Read the model definition and answer for the solid it produces. Units are mm, in the model's axes. Face numbers are marked on the shaded views. Give positions to 0.01 mm unless a question says otherwise; leave off trailing zeros. Loops run counter-clockwise (first coordinate to the right, second up) from the corner with the lowest first, then second, coordinate; pieces in that order, holes last.
(1) Determine the mould class of the marked faces 1 and 2 for opening direction X: pulls with the +X half, pulls with the -X half, needs draft (parallel to the pull), parting line crosses it, or undercut.
(2) Find section A-A, the plane x = 0. Write down the section's boundary in (y, z).
(3) Find section B-B, the plane y = 34. Write down the section's boundary in (x, z).
(4) Straight lines are drawn through the part: probe 1 along Y at (x, z) = (-5.5, 15.5); probe 2 along Y at (x, z) = (-3.5, -3); probe 3 along Y at (x, z) = (13, -24.5). For each, find the intervals that lie inside material, in ascending order.
(5) Each of these flat-tipped pins is pushed along its axis until it touches: P1, Ø10.5, axis at x = 6, z = 0, coming from the -Y side; P2, Ø3, axis at x = -19, y = -20.5, coming from the -Z side; P3, Ø6, axis at x = -2, y = 187.5, coming from the +Z side. Where does it stop, or does it pass through?
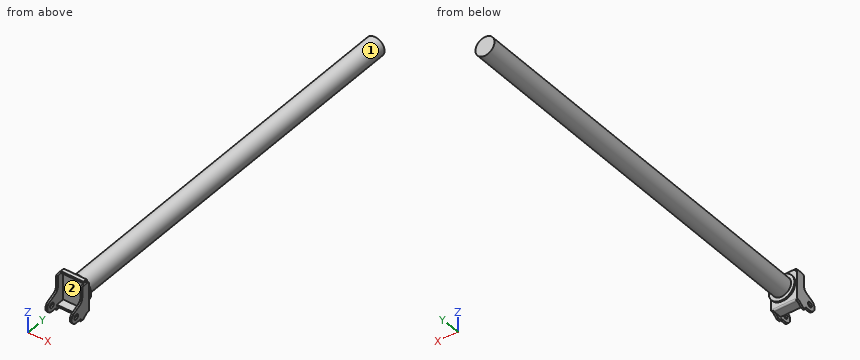
```python
from build123d import *

# Parameters (mm, degrees)
SKETCH1_W           = 35.2425
SKETCH1_H           = 45.085
BOSS_EXTRUDE1_DEPTH = 2.794
SKETCH3_W           = 35.2425
SKETCH3_H           = 7.62
BOSS_EXTRUDE2_DEPTH = 2.794
SKETCH4_W           = 35.2425
SKETCH4_H           = 15.875
BOSS_EXTRUDE3_DEPTH = 2.794
SKETCH5_R           = 3.99415
BOSS_EXTRUDE5_DEPTH = 2.794
SKETCH8_R           = 14.8209
BOSS_EXTRUDE6_DEPTH = 609.6
FILLET1_R           = 2.54


with BuildPart() as part:
    # Sketch1 → Boss-Extrude1 (new body)
    with BuildSketch(Plane(origin=(0, 0, 0), x_dir=(1, 0, 0), z_dir=(0, 1, 0))):
        Rectangle(SKETCH1_W, SKETCH1_H)
    extrude(amount=BOSS_EXTRUDE1_DEPTH)

    # Sketch3 → Boss-Extrude2 (add)
    with BuildSketch(Plane.XY.offset(22.5425)):
        with Locations((0, -1.016)):
            Rectangle(SKETCH3_W, SKETCH3_H)
    extrude(amount=BOSS_EXTRUDE2_DEPTH)

    # Sketch4 → Boss-Extrude3 (add)
    with BuildSketch(Plane(origin=(0, 0, -22.5425), x_dir=(-1, 0, 0), z_dir=(0, 0, -1))):
        with Locations((0, -5.1435)):
            Rectangle(SKETCH4_W, SKETCH4_H)
    extrude(amount=BOSS_EXTRUDE3_DEPTH)

    # Sketch5 → Boss-Extrude5 (add)
    with BuildSketch(Plane.ZY.offset(17.62125)):
        with BuildLine():
            Line((-24.5745, 2.794), (-24.5745, -0.249652205))
            ThreePointArc((-24.5745, -0.249652205), (-24.707295287, -1.060186269), (-25.091795645, -1.785968283))
            Line((-25.091795645, -1.785968283), (-30.3911, -8.763))
            Line((-30.3911, -8.763), (-30.3911, -13.843))
            Line((-30.3911, -13.843), (-26.9875, -13.843))
            Line((-26.9875, -13.843), (-26.9875, -23.3045))
            ThreePointArc((-26.9875, -23.3045), (-19.506235123, -32.571845213), (-8.869629771, -27.213147793))
            Line((-8.869629771, -27.213147793), (-4.188060723, -16.867828085))
            ThreePointArc((-4.188060723, -16.867828085), (-0.439339327, -12.518932794), (5.068277097, -10.8966))
            Line((5.068277097, -10.8966), (19.5707, -10.8966))
            ThreePointArc((19.5707, -10.8966), (21.366751224, -10.152651224), (22.1107, -8.3566))
            Line((22.1107, -8.3566), (22.1107, 0.254))
            ThreePointArc((22.1107, 0.254), (21.366751224, 2.050051224), (19.5707, 2.794))
            Line((19.5707, 2.794), (-24.5745, 2.794))
        make_face()
        with Locations((-17.50695, -23.3045)):
            Circle(SKETCH5_R, mode=Mode.SUBTRACT)
    boss_extrude5 = extrude(amount=BOSS_EXTRUDE5_DEPTH)

    # Mirror1: Boss-Extrude5 across plane
    add(boss_extrude5.mirror(Plane(origin=(0, 0, 0), x_dir=(0, 0, 1), z_dir=(1, 0, 0))))

    # Sketch6 → Revolve1 (revolve)
    with BuildSketch(Plane(origin=(0, 0, 0), x_dir=(0, 0, -1), z_dir=(1, 0, 0))):
        Polygon((0.5588, 2.794), (17.2339, 2.794), (17.2339, 6.1087), (20.5994, 6.1087), (20.5994, 8.1153), (0.5588, 8.1153), align=None)
    revolve(axis=Axis((0, 2.794, -0.5588), (0, 1, 0)))

    # Sketch8 → Boss-Extrude6 (add)
    with BuildSketch(Plane(origin=(0, 8.1153, 0), x_dir=(1, 0, 0), z_dir=(0, 1, 0))):
        with Locations(Location((0, 0, 0), (0, 0, 90))):
            Circle(SKETCH8_R)
    extrude(amount=BOSS_EXTRUDE6_DEPTH)

    # Fillet1
    fillet1_edges = [part.edges().sort_by_distance(p)[0] for p in [
        (0, 2.794, -25.3365),
        (0, 2.794, 25.3365),
    ]]
    fillet(fillet1_edges, radius=FILLET1_R)


solid = part.part
```
Entries:
1. face 1: parting line crosses it
1. face 2: undercut
2. outline: (-13.08, -25.34) - (0.25, -25.34) arc R2.54 ccw to (2.79, -22.8) - (2.79, -17.23) - (6.11, -17.23) - (6.11, -20.6) - (8.12, -20.6) - (8.12, -14.82) - (617.72, -14.82) - (617.72, 14.82) - (8.12, 14.82) - (8.12, 19.48) - (6.11, 19.48) - (6.11, 16.12) - (2.79, 16.12) - (2.79, 22.8) arc R2.54 ccw to (0.25, 25.34) - (-4.83, 25.34) - (-4.83, 22.54) - (0, 22.54) - (0, -22.54) - (-13.08, -22.54) - close
3. outline: circle Ø29.64 at (0, 0)
4. probe 1: y = 0 to 2.79, 6.11 to 8.12
4. probe 2: y = 0 to 617.72
4. probe 3: y = -13.08 to 2.14
5. P1: stops at y = 0
5. P2: stops at z = -26.99
5. P3: stops at z = 14.82
